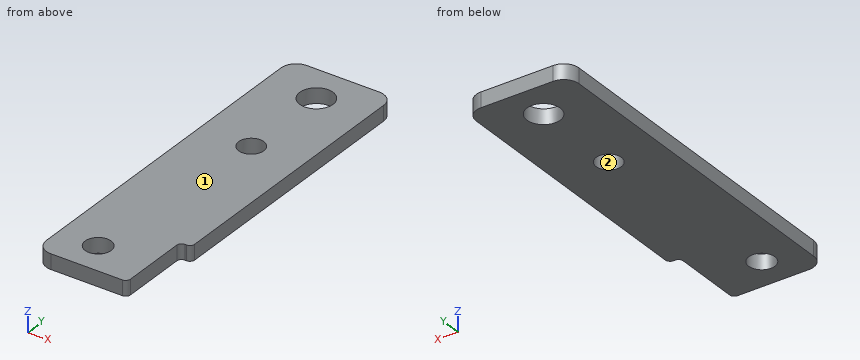
```python
from build123d import *

# Parameters (mm, degrees)
SKETCH1_R           = 3.5052
SKETCH1_R_2         = 2.75082
SKETCH1_R_3         = 2.654
BOSS_EXTRUDE1_DEPTH = 3.175
FILLET1_R           = 3.175
SKETCH3_W           = 2.54
SKETCH3_H           = 15.868015335
CUT_EXTRUDE2_DEPTH  = 47.655831395
FILLET2_R           = 1


with BuildPart() as part:
    # Sketch1 → Boss-Extrude1 (new body)
    with BuildSketch(Plane.XY):
        Polygon((-10.795, 31.115), (10.795, 31.115), (10.795, -31.115), (10.795, -45.278625787), (-10.795, -45.278625787), (-10.795, -31.115), align=None)
        with Locations((0, 23.1775)):
            Circle(SKETCH1_R, mode=Mode.SUBTRACT)
        with Locations((-2.4892, -38.41242)):
            Circle(SKETCH1_R_2, mode=Mode.SUBTRACT)
        with Locations((0, 3.734436212)):
            Circle(SKETCH1_R_3, mode=Mode.SUBTRACT)
    extrude(amount=BOSS_EXTRUDE1_DEPTH)

    # Fillet1
    fillet1_edges = [part.edges().sort_by_distance(p)[0] for p in [
        (10.795, -45.278625787, 1.5875),
        (-10.795, -45.278625787, 1.5875),
        (-10.795, 31.115, 1.5875),
        (10.795, 31.115, 1.5875),
    ]]
    fillet(fillet1_edges, radius=FILLET1_R)

    # Sketch3 → Cut-Extrude2 (cut, through all)
    with BuildSketch(Plane.XY.offset(3.175)):
        with Locations((9.706042249, -37.379761593)):
            Rectangle(SKETCH3_W, SKETCH3_H)
    extrude(amount=-CUT_EXTRUDE2_DEPTH, mode=Mode.SUBTRACT)

    # Fillet2
    fillet2_edges = [part.edges().sort_by_distance(p)[0] for p in [
        (10.795, -29.445753925, 1.5875),
        (8.436042249, -29.445753925, 1.5875),
        (8.436042249, -45.171964108, 1.5875),
    ]]
    fillet(fillet2_edges, radius=FILLET2_R)


solid = part.part
```
Work out the finished part from the listing and answer in its coordinate system (mm). Face numbers are marked on the shaded views. Round coordinates to 2 decimals unless told otherwise and drop trailing zeros. Write each loop counter-clockwise with the first axis right and the second up, starting at its lowest first coordinate (ties: lowest second). Pieces come first, ordered by that corner, then holes. Notation, with made-up numbers: (86, 89.25) - (129, 89.25) arc R12 cw to (129, 110.25) - close; hole circle Ø10 at (55.25, -16). An arc over 180 degrees is marked (long way). Return JSON: item names as keys, results as strings. Group by question number.
Q1. Each of these flat-tipped pins is pushed along its axis until it touches: pin 1 Ø1.6 at (y, z) = (-39, 1.5) entering from +X; pin 2 Ø4 at (x, y) = (6.5, 1.5) entering from -Z. Where does it stop, or does it pass through?
Q2. Find the intervals of material crossed by L1, parallel to Y at x = 0, z = 1.2 (3 decimals); L2, parallel to X at y = 21, z = 2.4 (3 decimals); L3, parallel to X at y = 24, z = 1.4 (3 decimals), in increasing order.
Q3. The mould has two halves that part along X. Classify the marked faces 1 and 2: released by +X, released by -X, zero draft, split by the parting line, or undercut.
Q4. The part is cut by section A-A on x = 1.75. Write down the section's boundary in (y, z) (3 decimals), then the cut area to 3 significant figures.
Q5. The part is cut by section B-B on z = 0.95. Count the separate pieces of the cut face and the enclosed holes in it, then the cut area to 3 significant figures.
Solved:
{
 "1": {"pin 1": "x = 8.44", "pin 2": "z = 0"},
 "2": {"L1": "-45.279 to -39.583, -37.242 to 1.08, 6.388 to 19.672, 26.683 to 31.115", "L2": "-10.795 to -2.747, 2.747 to 10.795", "L3": "-10.795 to -3.407, 3.407 to 10.795"},
 "3": {"face 1": "zero draft", "face 2": "undercut"},
 "4": {"outline": "(-45.279, 0) - (1.739, 0) - (1.739, 3.175) - (-45.279, 3.175) - close; (5.73, 0) - (20.14, 0) - (20.14, 3.175) - (5.73, 3.175) - close; (26.215, 0) - (31.115, 0) - (31.115, 3.175) - (26.215, 3.175) - close", "area": "211 mm²"},
 "5": {"separate pieces": "1", "enclosed holes": "3", "area": "1,520 mm²"}
}
